Geometry: final body of the model. Coordinates: model frame, mm. Give positions to 0.01 mm unless a question says otherwise; leave off trailing zeros. Order: outer loops, then holes, each group sorted by start corner. A loop starts at its lowest first (then second) coordinate and runs counter-clockwise, first axis right, second up. Notation, with made-up numbers: (17, 7) - (25, 7) arc R10 cw to (25, 25) - close; hole circle Ø8 at (-24, 33.5). An arc over 180 degrees is marked (long way). Put each result on its own line as item: value. Start each with the question number.
1. Section A-A on x = 0.95. Return the cut outline in (y, z), plus the area to 3 significant figures.
2. Section C-C on y = 1182.5. Return the cut outline in (x, z), plus the area to 3 significant figures.
3. First-contact query: P1, Ø2, axis at y = 1514.5, z = -144.5, coming from the -X side; P2, Ø1.5, axis at x = 1.5, z = -197.5, coming from the +Y side; P3, Ø1.5, axis at x = 1.5, y = 1519, coming from the -Z side; P4, Ø1, axis at x = 0.5, y = 1164, coming from the -Z side. Flat tips, straight axial feed; report the tip coordinate or a pass-through.
4. Section D-D on y = 1539. Return the cut outline in (x, z).
5. Ray query, line 1 along Y through (x, z) = (1.25, -133.5); line 2 along Z through (x, y) = (0.7, 1482.5); line 3 along Y through (x, z) = (0.8, -25). Return the intervals inside material, ascending. Write a range as from..to.
from build123d import *

# Parameters (mm, degrees)
BOSS_EXTRUDE1_DEPTH = 5.08
SKETCH11_W          = 41.321018404
SKETCH11_H          = 82.171066474
SKETCH11_W_2        = 64.858701062
SKETCH11_H_2        = 131.277002868
CUT_EXTRUDE1_DEPTH  = 1593.302629235


with BuildPart() as part:
    # Sketch5 → Boss-Extrude1 (new body)
    with BuildSketch(Plane(origin=(0, 0, 0), x_dir=(0, 0, -1), z_dir=(1, 0, 0))):
        Polygon((-1.661660189, 1095.375698265), (212.544479643, 1095.145979446), (213.062028944, 1577.745701931), (-1.144110888, 1577.97542075), align=None)
    extrude(amount=BOSS_EXTRUDE1_DEPTH)

    # Sketch11 → Cut-Extrude1 (cut, through all)
    with BuildSketch(Plane(origin=(5.08, 0, 0), x_dir=(0, 0, -1), z_dir=(1, 0, 0))):
        with Locations((192.401519742, 1536.660168694)):
            Rectangle(SKETCH11_W, SKETCH11_H)
        with Locations((212.838086125, 1126.439608027)):
            Rectangle(SKETCH11_W_2, SKETCH11_H_2)
    extrude(amount=-CUT_EXTRUDE1_DEPTH, mode=Mode.SUBTRACT)


solid = part.part
Resolved:
1. outline: (1095.18, -180.41) - (1192.08, -180.41) - (1192.08, -212.65) - (1495.57, -212.97) - (1495.57, -171.74) - (1577.75, -171.74) - (1577.75, -213.06) - (1577.98, 1.14) - (1095.38, 1.66) - close
1. area: 96,900 mm^2
2. outline: (0, -180.41) - (5.08, -180.41) - (5.08, 1.57) - (0, 1.57) - close
2. area: 924 mm^2
3. P1: x = 0
3. P2: y = 1577.76
3. P3: z = -171.74
3. P4: z = -180.41
4. outline: (0, -171.74) - (5.08, -171.74) - (5.08, 1.19) - (0, 1.19) - close
5. line 1: 1095.23..1577.83
5. line 2: -212.96..1.25
5. line 3: 1095.35..1577.95
